Can you work these out from the model? Positions are in its coordinate system, mm. A direction names the side the tool comes from. Round coordinates to 2 decimals unless told otherwise and drop trailing zeros. Loops run counter-clockwise (first coordinate to the right, second up) from the corner with the lowest first, then second, coordinate; pieces in that order, holes last. Notation, with made-up numbers: (85, 89.5) - (120, 89.5) arc R24 cw to (120, 128.5) - close; hole circle Ø7 at (14.5, 1). An arc over 180 degrees is marked (long way). Answer as CSV lines item,"result".
```python
from build123d import *

# Parameters (mm, degrees)
EXTRUDE_1_DEPTH     = 76
EXTRUDE_2_REACH     = 182.051
SKETCH_2_R          = 9.5
SKETCH_3_R          = 3.25
CUT_EXTRUDE_1_DEPTH = 76
SKETCH_4_R          = 6.5
CUT_EXTRUDE_2_DEPTH = 76
FILLET_2_R          = 19


with BuildPart() as part:
    # 스케치1 → 보스-돌출1 (new body)
    with BuildSketch(Plane.XY):
        Polygon((0, 0), (152, 0), (152, -51), (133, -51), (133, -19), (0, -19), align=None)
    extrude(amount=EXTRUDE_1_DEPTH)

    # 보스-돌출2: up to this face of the body (flat: up to its plane)
    extrude_2_end = Plane(part.part.faces().sort_by_distance((76, 0, 38))[0])
    # 스케치2 → 보스-돌출2 (add, up to the picked face)
    with BuildSketch(Plane(origin=(114, 65.817930688, 0), x_dir=(0, 0, -1), z_dir=(0.8660254037844398, 0.499999999999998, 0)), mode=Mode.PRIVATE) as extrude_2_sk1:
        with BuildLine():
            Line((-61.604391893, -46), (-61.604391893, -76))
            Line((-61.604391893, -76), (-17.604391893, -76))
            Line((-17.604391893, -76), (-17.604391893, -46))
            ThreePointArc((-17.604391893, -46), (-39.604391893, -24), (-61.604391893, -46))
        make_face()
        with Locations(Location((-39.604391893, -46, 0), (0, 0, 90))):
            Circle(SKETCH_2_R, mode=Mode.SUBTRACT)
    extrude_2_tool1 = split(extrude(extrude_2_sk1.sketch, amount=-EXTRUDE_2_REACH, mode=Mode.PRIVATE), bisect_by=extrude_2_end, keep=Keep.BOTH, mode=Mode.PRIVATE)
    add(extrude_2_tool1.solids().sort_by(Axis((144.5, 12.990381, 60.923216), (-0.8660254037844398, -0.499999999999998, 0)))[0])

    # 스케치3 → 컷-돌출1 (cut)
    with BuildSketch(Plane(origin=(152, 0, 0), x_dir=(0, 0, -1), z_dir=(1, 0, 0))):
        with Locations((-57.45899172, -35.913585608)):
            Circle(SKETCH_3_R)
        with Locations((-19.45899172, -35.913585608)):
            Circle(SKETCH_3_R)
    extrude(amount=-CUT_EXTRUDE_1_DEPTH, mode=Mode.SUBTRACT)

    # 스케치4 → 컷-돌출2 (cut)
    with BuildSketch(Plane(origin=(0, 0, 0), x_dir=(1, 0, 0), z_dir=(0, 1, 0))):
        with Locations(Location((15.665320211, -57, 0), (0, 0, 270))):
            Circle(SKETCH_4_R)
        with Locations(Location((15.665320211, -19, 0), (0, 0, 270))):
            Circle(SKETCH_4_R)
    extrude(amount=-CUT_EXTRUDE_2_DEPTH, mode=Mode.SUBTRACT)

    # 필렛2
    fillet_2_edges = [part.edges().sort_by_distance(p)[0] for p in [
        (142.5, -51, 76),
        (142.5, -51, 0),
    ]]
    fillet(fillet_2_edges, radius=FILLET_2_R)


solid = part.part
```
Q1. Imagine slicing it at C-C (z = 5.5). Write out the boundary of the cut face in (x, y).
Checks:
outline,"(0, -19) - (133, -19) - (133, -45.37) - (152, -45.37) - (152, 0) - (0, 0) - close"
Q2. I'm going to push flat-ended pins straight in: pin 1 Ø8 at (x, y) = (122.5, 12.5) entering from -Z; pin 2 Ø8 at (y, z) = (10.5, 51.5) entering from +X; pin 3 Ø4 at (x, z) = (27.5, 31.5) entering from -Y. Where does each tip first touch, or does it pass through?
Checks:
pin 1,"z = 17.6"
pin 2,"x = 148.25"
pin 3,"y = -19"
Q3. Imagine slicing it at B-B (y = -8). Write out the boundary of the cut face in (x, z).
Checks:
outline,"(0, 0) - (152, 0) - (152, 76) - (0, 76) - close; hole circle Ø13 at (15.67, 19); hole circle Ø13 at (15.67, 57)"
Q4. If I drill on line 1 along X through (y, z) = (-10, 19); line 2 along Y through (x, z) = (36, 53); line 3 along X through (y, z) = (12.5, 42), over which ranges is the centre line in solid material (lowest first)? Write a range as [from, to].
Checks:
line 1,"[0, 9.17], [22.17, 152]"
line 2,"[-19, 0]"
line 3,"[69.91, 95.26], [132.04, 144.78]"
Q5. Imagine slicing it at A-A (z = 52.5). Write out the boundary of the cut face in (x, y), then the cut area to 3 significant figures.
Checks:
outline,"(0, -19) - (10.97, -19) - (10.97, 0) - (0, 0) - close; (20.36, -19) - (133, -19) - (133, -51) - (152, -51) - (152, 0) - (128.09, 41.42) - (56.35, 0) - (20.36, 0) - close"
area,"5,300 mm²"
Q6. We'd pull the mould along Z, two halves only. Please class faces 4 (the cylindrical face through (15.951, -9.367, 12.506)), 5 (the flat face through (129, 12, 17.604)), 6 (the flat face through (141.707, 17.828, 35.024)), 7 (the flat face through (77, -9, 76)): pulls with the +Z half, pulls with the -Z half, needs draft (parallel to the pull), parting line crosses it, or undercut.
Checks:
face 4,"undercut"
face 5,"pulls with the -Z half"
face 6,"needs draft"
face 7,"pulls with the +Z half"
Q7. On a 3-axis mill with a long thin cutter (end or side, diameter ignored), from which of +Z, -Z, +X, -X, +Y, -Y can I reach the whole of each face in a straight line? I mean faces 1 (the flat face through (67, -19, 37)), 2 (the flat face through (58, 0, 21)), 3 (the flat face through (126, 6, 61.604)). Say none if no direction works.
Checks:
face 1,"+Z, -Z, -X, -Y"
face 2,"-X, +Y"
face 3,"+Z, +X, -X, +Y"
